Autodesk Fusion 360 part; units mm, degrees
sketch "Esquisse1" plane through (0, 0, 0) normal (1, 0, 0) x (0, 1, 0)
  line L0 (-50, 85) -> (50, 85)
  line L1 (50, 85) -> (50, 0)
  line L2 (50, 0) -> (-50, 0)
  line L3 (-50, 0) -> (-50, 85)
  line L4 (0, 1.75) -> (0, 22.5)
  dimension "d1" = 85
  dimension "d2" = 100
extrude "Extrusion1" add sketch "Esquisse1" along normal blind 30
sketch "Esquisse2" plane through (0, 0, 0) normal (-1, 0, 0) x (0, -1, 0)
  line L0 (-50, 0) -> (50, 0)
  line L1 (50, 0) -> (50, 85)
  line L2 (50, 85) -> (-50, 85)
  line L3 (-50, 85) -> (-50, 0)
  circle A0 centre (-35, 72.5) radius 4.075
  line L4 (0, 1.75) -> (0, 22.5)
  dimension "d5" = 8.15
  dimension "d6" = 12.5
  dimension "d7" = 35
extrude "Extrusion2" cut sketch "Esquisse2" against normal blind 40 contours A0
mirror "Symétrie miroir1" about plane through (0, 0, 0) normal (0, 1, 0) of "Extrusion2"
equation "d7 = ( 70 / 2 ) * 1 mm"
Geometry check sheet. Reference: the model listing, model coordinates, mm. Give positions to 0.01 mm unless a question says otherwise; leave off trailing zeros. Order: outer loops, then holes, each group sorted by start corner. A loop starts at its lowest first (then second) coordinate and runs counter-clockwise, first axis right, second up.
1) Material ranges on probe 1 along Z at (x, y) = (23.25, -35) (3 decimals); probe 2 along Z at (x, y) = (17.75, -38), recorded low to high.
Results are:
probe 1: z = 0 to 68.425, 76.575 to 85
probe 2: z = 0 to 69.74, 75.26 to 85
2) Cross-section at A-A (y = 35). Record the boundary of the cut face in (x, z) (3 decimals).
Results are:
outline: (0, 0) - (30, 0) - (30, 68.425) - (0, 68.425) - close; (0, 76.575) - (30, 76.575) - (30, 85) - (0, 85) - close
3) Draft check along Z on faces 1 (the flat face through (15, -1, 85)), 2 (the cylindrical face through (14.79, 33.12, 68.885)), 3 (the flat face through (30, -1, 43)), 4 (the cylindrical face through (14.79, -33.12, 76.115)). Enter one of: released by +Z, released by -Z, zero draft, split by the parting line, or undercut.
Results are:
face 1: released by +Z
face 2: undercut
face 3: zero draft
face 4: undercut
4) Cross-section at B-B (z = 72.5). Record the boundary of the cut face in (x, y) (3 decimals), then the cut area to 3 significant figures.
Results are:
outline: (0, -50) - (30, -50) - (30, -39.075) - (0, -39.075) - close; (0, -30.925) - (30, -30.925) - (30, 30.925) - (0, 30.925) - close; (0, 39.075) - (30, 39.075) - (30, 50) - (0, 50) - close
area: 2,510 mm2
5) Gauge pin test, flat end, axial feed: pin 1 (7.5 mm diameter, centred on y = 35, z = 72.5, fed in from +X) (1 decimal). Record the tip position at first contact, or that the pin passes through.
Results are:
pin 1: passes through
